```python
from build123d import *

# Parameters (mm, degrees)
BOSS_EXTRUDE1_DEPTH = 46
SKETCH1_3_R         = 23.5
BOSS_EXTRUDE2_DEPTH = 50


with BuildPart() as part:
    # Sketch1 → Boss-Extrude1 (new body)
    with BuildSketch(Plane(origin=(0, 0, 0), x_dir=(1, 0, 0), z_dir=(0, 1, 0))):
        with BuildLine():
            ThreePointArc((18.072726342, -15.020870899), (0, -23.5), (-18.072726342, -15.020870899))
            Line((-18.072726342, -15.020870899), (-14.925557853, -46.492555785))
            ThreePointArc((-14.925557853, -46.492555785), (0, -60), (14.925557853, -46.492555785))
            Line((14.925557853, -46.492555785), (18.072726342, -15.020870899))
        make_face()
    extrude(amount=-BOSS_EXTRUDE1_DEPTH)

    # Sketch1_3 → Boss-Extrude2 (add)
    with BuildSketch(Plane(origin=(0, 0, 0), x_dir=(1, 0, 0), z_dir=(0, 1, 0))):
        with Locations(Location((0, 0, 0), (0, 0, 270))):
            Circle(SKETCH1_3_R)
    extrude(amount=-BOSS_EXTRUDE2_DEPTH)

    # Sketch2 → Revolve1 (revolve)
    with BuildSketch(Plane(origin=(0, -28, 0), x_dir=(1, 0, 0), z_dir=(0, 1, 0)), mode=Mode.PRIVATE) as revolve1_sk:
        Polygon((-19.721704902, 12.779059268), (0, 12.779059268), (0, 55), (-16, 55), align=None)
    revolve(revolve1_sk.sketch.rotate(Axis((0, -28, 0), (0, 0, -1)), 180), axis=Axis((0, -28, 0), (0, 0, -1)))


solid = part.part
```
Design review of the part built by this model. Coordinates are the model's own, in mm. A direction names the side the tool comes from. Coordinates: 2 decimals unless noted, no trailing zeros. Order: outer loops, then holes, each group sorted by start corner. A loop starts at its lowest first (then second) coordinate and runs counter-clockwise, first axis right, second up.
1) Take a section at B-B, the plane z = -19. Give the boundary of the cut face in (x, y), and give its area (3 significant figures).
2) Wall thickness on line 1 along Y through (x, z) = (0, 50.5); line 2 along X through (y, z) = (-37, 11); line 3 along Y through (x, z) = (7, -34.5): over which ranges is each line inside the solid? List them lowest first.
3) Take a section at A-A, the plane x = 0. Give the boundary of the cut face in (y, z), and give its area (3 significant figures).
4) For faces 1 (the cylindrical face through (23.3, -24.65, -3.06)), 2 (the flat face through (16.477, -22.678, 30.977)), list the 3-axis set-ups (+Z, -Z, +X, -X, +Y, -Y) from which the entire face can be reached by the end or side of a thin tool; tool diameter is ignored.
5) Clearance check with flat-ended pins moving along their axes: pin 1 (12 mm diameter, centred on x = 14.5, z = 47.5, fed in from -Y); pin 2 (8 mm diameter, centred on y = -25, z = 7, fed in from -X); pin 3 (5 mm diameter, centred on x = -14.5, y = -26.5, fed in from +Z). State where each tip first meets the part, or that it passes through.
6) Take a section at C-C, the plane y = -8. Give the boundary of the cut face in (x, z).
Returned:
1. outline: (-13.83, -50) - (13.83, -50) - (13.83, -41.28) arc R19.17 ccw to (13.83, -14.72) - (13.83, 0) - (-13.83, 0) - (-13.83, -14.72) arc R19.17 ccw to (-13.83, -41.28) - close
1. area: 1,580 mm2
2. line 1: y = -46 to 0
2. line 2: x = -20.77 to 20.77
2. line 3: y = -44.37 to -11.63
3. outline: (-50, -23.5) - (-46.78, -23.5) - (-44, -55) - (-12, -55) - (-9.22, -23.5) - (0, -23.5) - (0, 60) - (-46, 60) - (-46, 23.5) - (-50, 23.5) - close
3. area: 5,120 mm2
4. face 1: none
4. face 2: +Z, +X, +Y, -Y
5. pin 1: stops at y = -46
5. pin 2: stops at x = -23.31
5. pin 3: stops at z = 54
6. outline: (-18.07, 15.02) arc R23.5 ccw (long way) to (18.07, 15.02) - (14.93, 46.49) arc R15 ccw to (-14.93, 46.49) - close
